Part model, mm, in its own coordinate system. A direction names the side the tool comes from. Round coordinates to 2 decimals unless told otherwise and drop trailing zeros. Loops run counter-clockwise (first coordinate to the right, second up) from the corner with the lowest first, then second, coordinate; pieces in that order, holes last. Notation, with made-up numbers: M 29,50 L 57,50 A29 ccw 57,73 Z; hole C 77.25,59 d3. An arc over 180 degrees is marked long. Put each result on its own line as item: value. Start each with the question number.
1) Which spindle directions (+Z, -Z, +X, -X, +Y, -Y) get a long thin tool onto all of the face, cutting with end or side? Do faces 1 (the flat face through (-21, 0, -38)), 2 (the cylindrical face through (2.835, 13.311, 42.906)). Say none if no direction does.
2) Pull direction X, two halves, no side cores. Call faces 3 (the cylindrical face through (-44.83, 3.45, -14.12)), 4 (the cylindrical face through (-14.845, 4.591, 42.446)), 5 (the cylindrical face through (44.96, 4.7, 0.27)): +X half, -X half, draft (parallel to the pull), parting line (faces both ways), or undercut.
3) Slice it at C-C on y = 18.75. Give the cut face in (x, z), then the cut area to 3 significant figures.
4) Slice it at B-B on y = 3.5. Give the cut face in (x, z), then the cut area to 3 significant figures.
5) Slice it at D-D on z = -38. Give the cut face in (x, y).
6) Drop flat-ended pins along their axis: pin 1 Ø6 at (x, y) = (2, 16) entering from +Z; pin 2 Ø3 at (x, y) = (-32.5, 4.5) entering from +Z; pin 3 Ø4 at (y, z) = (16, -24) entering from +X. Give the stop position or say it passes through.
7) Probe line 1 along Z through (x, y) = (0, 27.7); line 2 along Z through (x, y) = (0, 12); line 3 along Y through (x, z) = (14.5, -9). List the from-to ranges inside material, lowest first.
Autodesk Inventor part; units mm, degrees
ref_plane "Work Plane2" through (47, 0, 0) normal (1, 0, 0) x (0, 1, 0)
ref_plane "XZ Plane" through (0, 0, 0) normal (0, 1, 0) x (-1, 0, 0)
ref_plane "XY Plane" through (0, 0, 0) normal (0, 0, 1) x (1, 0, 0)
sketch "Sketch1" plane through (0, 0, 0) normal (0, 1, 0) x (-1, 0, 0)
  circle A0 centre (0, 0) radius 47
  circle A1 centre (0, 0) radius 43
  dimension "d0" = 94
  dimension "d8" = 4
extrude "Extrusion1" add sketch "Sketch1" along normal blind 7
sketch "Sketch2" plane through (0, 7, 0) normal (0, 1, 0) x (1, 0, 0)
  circle A0 centre (0, 0) radius 43
  circle A1 centre (0, 0) radius 48
  dimension "d38" = 86
  dimension "d39" = 96
extrude "Extrusion2" add sketch "Sketch2" along normal blind 20
sketch "Sketch6" plane through (0, 27, 0) normal (0, 1, 0) x (1, 0, 0)
  circle A0 centre (0, 0) radius 48
extrude "Extrusion5" add sketch "Sketch6" along normal blind 2
ref_plane "Work Plane2" through (47, 0, 0) normal (1, 0, 0) x (0, 1, 0)
sketch "Sketch7" plane through (47, 0, 0) normal (1, 0, 0) x (0, 1, 0)
  point P0 (0, 0)
  point P1 (3.5, 0)
hole "Hole1" at (47, 3.5, 0) direction (-1, 0, 0) diameter 2.459 depth 5
pattern_circular "Circular Pattern6" count 3 over 220 about axis through (0, 0, 0) along (0, 1, 0) of "Hole1" both ways yes
sketch "Sketch8" plane through (0, 29, 0) normal (0, 1, 0) x (1, 0, 0)
  circle A0 centre (0, -30) radius 1.55
  point P0 (0, 0)
  dimension "d62" = 3.1
extrude "Extrusion6" cut sketch "Sketch8" against normal blind 2
properties part number "Abdeckung_Gaseinlass_new"
Recorded:
1. face 1: +Z, -Z, +X, -X, -Y
1. face 2: -Y
2. face 3: parting line
2. face 4: undercut
2. face 5: draft
3. outline: C 0,0 d96; hole C 0,0 d86
3. area: 1,430 mm2
4. outline: M -17.22,-43.73 L -15.86,-39.97 A43 cw -15.86,39.97 L -17.22,43.73 A47 ccw Z; M -14.91,-44.57 A47 ccw 46.98,-1.23 L 42.98,-1.23 A43 cw -13.55,-40.81 Z; M -14.91,44.57 L -13.55,40.81 A43 cw 42.98,1.23 L 46.98,1.23 A47 ccw Z
4. area: 1,100 mm2
5. outline: M -29.33,7 L -27.66,7 L -27.66,0 L -20.12,0 L -20.12,27 L 20.12,27 L 20.12,0 L 27.66,0 L 27.66,7 L 29.33,7 L 29.33,29 L -29.33,29 Z
6. pin 1: stops at z = 48
6. pin 2: stops at z = 35.33
6. pin 3: stops at x = 42.66
7. line 1: z = -48 to 28.45, 31.55 to 48
7. line 2: z = -48 to -43, 43 to 48
7. line 3: y = 27 to 29
